from build123d import *

# Parameters (mm, degrees)
BOSS_EXTRUDE1_DEPTH   = 7.9375
F_8_CLEARANCE_HOLE1_D = 4.9149
F_8_CLEARANCE_HOLE2_D = 4.9149
SKETCH7_R             = 5.08
CUT_EXTRUDE1_DEPTH    = 2.032
FILLET1_R             = 1.5875
CHAMFER2_SIZE         = 1.27


with BuildPart() as part:
    # Sketch2 → Boss-Extrude1 (new body)
    with BuildSketch(Plane.XY):
        with BuildLine():
            Line((-9.525, 42.96918), (-9.525, 0))
            ThreePointArc((-9.525, 0), (0, -9.525), (9.525, 0))
            Line((9.525, 0), (9.525, 33.44418))
            ThreePointArc((9.525, 33.44418), (6.735192091, 40.179372091), (0, 42.96918))
            Line((0, 42.96918), (-9.525, 42.96918))
        make_face()
    extrude(amount=BOSS_EXTRUDE1_DEPTH)

    # #8 Clearance Hole1 (through all)
    with Locations(Plane.XY.offset(7.9375)):
        with Locations((0, 0)):
            Hole(F_8_CLEARANCE_HOLE1_D / 2)

    # #8 Clearance Hole2 (through all)
    with Locations(Plane.XY.offset(7.9375)):
        with Locations((0, 33.44418)):
            Hole(F_8_CLEARANCE_HOLE2_D / 2)

    # Sketch7 → Cut-Extrude1 (cut)
    with BuildSketch(Plane(origin=(0, 0, 0), x_dir=(-1, 0, 0), z_dir=(0, 0, -1))):
        with Locations((0, 33.44418)):
            Circle(SKETCH7_R)
    extrude(amount=-CUT_EXTRUDE1_DEPTH, mode=Mode.SUBTRACT)

    # Fillet1
    fillet1_edges = [part.edges().sort_by_distance(p)[0] for p in [
        (-9.525, 42.96918, 3.96875),
    ]]
    fillet(fillet1_edges, radius=FILLET1_R)

    # Chamfer2
    chamfer2_edges = [part.edges().sort_by_distance(p)[0] for p in [
        (6.735192091, 40.179372091, 7.9375),
        (-3.96875, 42.96918, 7.9375),
        (-9.525, 20.69084, 0),
        (-9.525, 20.69084, 7.9375),
        (-9.060032015, 42.504212015, 0),
        (-9.060032015, 42.504212015, 7.9375),
        (0, -9.525, 7.9375),
        (-3.96875, 42.96918, 0),
        (6.735192091, 40.179372091, 0),
        (9.525, 16.72209, 0),
        (0, -9.525, 0),
        (9.525, 16.72209, 7.9375),
    ]]
    chamfer(chamfer2_edges, length=CHAMFER2_SIZE)


solid = part.part
Geometry: final body of the model. Coordinates: model frame, mm. Round coordinates to 2 decimals unless told otherwise and drop trailing zeros. Loops run counter-clockwise (first coordinate to the right, second up) from the corner with the lowest first, then second, coordinate; pieces in that order, holes last. Notation, with made-up numbers: M 12,16 L 47,16 A24 cw 47,43 Z; hole C 47.5,29 d4. An arc over 180 degrees is marked long. Put each result on its own line as item: value. Start each with the question number.
(1) Material intervals for line 1 along Y through (x, z) = (0, 5.75) (3 decimals); line 2 along Y through (x, z) = (-0.25, 7); line 3 along Z through (x, y) = (-3, 37.5), sorted ascending. Write a range as [from, to].
(2) Contact query for flat-ended pins moving along their axis: pin 1 Ø1.5 at (x, z) = (3, 6.5) entering from -Y; pin 2 Ø2 at (x, z) = (7.5, 7) entering from +Y; pin 3 Ø3 at (x, y) = (0, 31.5) entering from -Z. Output: stop coordinate, or through.
(3) Section query A-A (z = 4.75). State how many separate pieces and enclosed holes the cut face has, then the cut area to 3 significant figures.
(4) Section query B-B (y = 19). Return loops of the section in (x, z) (1 decimal), then the cut area to 3 significant figures.
(5) Section query C-C (z = 7.25). Return loops of the section in (x, y) (1 decimal), then the cut area to 3 significant figures.
(6) Draft query along Y for faces 1 (the face through (-0.19, -8.47, 7.72)), 2 (the face through (1, 31, 2.032)), 3 (the face through (6.059, 39.371, 7.717)). Return one class per face: +Y half, -Y half, draft (parallel to the pull), parting line (faces both ways), or undercut.
Findings below:
1. line 1: y = [-9.525, -2.457], [2.457, 30.987], [35.902, 42.969]
1. line 2: y = [-9.19, -2.44], [2.44, 31], [35.89, 42.64]
1. line 3: z = [2.03, 7.94]
2. pin 1: stops at y = -9.26
2. pin 2: stops at y = 40.35
2. pin 3: stops at z = 2.03
3. separate pieces: 1
3. enclosed holes: 2
3. area: 903 mm2
4. outline: M -9.5,1.3 L -8.3,0 L 8.3,0 L 9.5,1.3 L 9.5,6.7 L 8.3,7.9 L -8.3,7.9 L -9.5,6.7 Z
4. area: 148 mm2
5. outline: M -8.9,0 A8.9 ccw 8.9,0 L 8.9,33.4 A8.9 ccw 0,42.4 L -7.9,42.4 A1 ccw -8.9,41.4 Z; hole C 0,0 d4.9; hole C 0,33.4 d4.9
5. area: 828 mm2
6. face 1: -Y half
6. face 2: undercut
6. face 3: +Y half
